Can you work these out from the model? Positions are in its coordinate system, mm. Face numbers are marked on the shaded views. Give positions to 0.01 mm unless a question says otherwise; leave off trailing zeros. Write each loop counter-clockwise with the first axis right and the second up, starting at its lowest first coordinate (ties: lowest second). Pieces come first, ordered by that corner, then holes.
1. Suppose I cut it at C-C (y = 11). Please give me the cut outline in (x, z) (1 decimal).
2. I'm going to push flat-ended pins straight in: pin 1 (12 mm diameter, centred on x = -8.5, y = -8.5, fed in from +Z); pin 2 (3 mm diameter, centred on y = 8.5, z = 13.5, fed in from -X); pin 3 (1.5 mm diameter, centred on x = 19.5, y = -7, fed in from -Z) (3 decimals). Where does each tip first touch, or does it pass through?
3. Thinking about a two-plate mould opening in X: for the marked faces 1, 2 and 3, which applies, pulls with the +X half, pulls with the -X half, needs draft (parallel to the pull), parting line crosses it, or undercut?
4. If I drill on probe 1 along Z at (x, y) = (-4, 0.75); probe 2 along X at (y, z) = (4.75, 0); probe 3 along Z at (x, y) = (-7, 7), over which ranges is the centre line in solid material (lowest first)?
5. Suppose I cut it at B-B (x = 0). Please give me the cut outline in (y, z), and give its area (3 significant figures).
6. Suppose I cut it at D-D (y = 7.75). Please give me the cut outline in (x, z) (1 decimal).
7. Suppose I cut it at A-A (z = 0). Please give me the cut outline in (x, y), and give its area (3 significant figures).
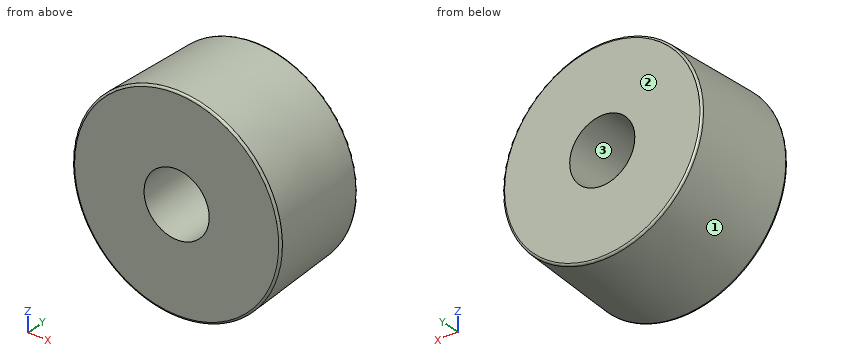
```python
from build123d import *

# Parameters (mm, degrees)
SKETCH1_R           = 25.4
SKETCH1_R_2         = 7.9375
BOSS_EXTRUDE1_DEPTH = 12.7
CHAMFER1_SIZE       = 25.4
CHAMFER1_SIZE_2     = 1.10898795
FILLET1_R           = 0.5


with BuildPart() as part:
    # Sketch1 → Boss-Extrude1 (new, symmetric)
    with BuildSketch(Plane(origin=(0, 0, 0), x_dir=(1, 0, 0), z_dir=(0, 1, 0))):
        with Locations(Location((0, 0, 0), (0, 0, 270))):
            Circle(SKETCH1_R)
        with Locations(Location((0, 0, 0), (0, 0, 270))):
            Circle(SKETCH1_R_2, mode=Mode.SUBTRACT)
    extrude(amount=BOSS_EXTRUDE1_DEPTH, both=True)

    # Chamfer1
    # the kernel refuses this chamfer: 25.4, 1.10898795 mm, written as the material it takes off along each edge
    with BuildSketch(Plane(origin=(0, 12.7, 0), x_dir=(0, 0, 1), z_dir=(-1, 0, 0))) as chamfer1_piece_1:
        Polygon((25.4, -CHAMFER1_SIZE), (25.4 - CHAMFER1_SIZE_2, 0), (25.4, 0), align=None)
    revolve(axis=Axis((0, 12.7, 0), (0, 1, 0)), mode=Mode.SUBTRACT)

    # Fillet1
    fillet1_edges = [part.edges().sort_by_distance(p)[0] for p in [
        (0, -12.7, -25.4),
        (0, 12.7, -24.29101205),
    ]]
    fillet(fillet1_edges, radius=FILLET1_R)


solid = part.part
```
Checks:
1. outline: circle Ø48.7 at (0, 0); hole circle Ø15.9 at (0, 0)
2. pin 1: stops at z = 25.14
2. pin 2: stops at x = -21.33
2. pin 3: stops at z = -16.765
3. face 1: parting line crosses it
3. face 2: needs draft
3. face 3: undercut
4. probe 1: z = -24.49 to -6.86, 6.86 to 24.49
4. probe 2: x = -24.64 to -7.94, 7.94 to 24.64
4. probe 3: z = -23.52 to -3.74, 3.74 to 23.52
5. outline: (-12.7, -24.88) arc R0.5 ccw to (-12.18, -25.38) - (12.22, -24.31) arc R0.5 ccw to (12.7, -23.81) - (12.7, -7.94) - (-12.7, -7.94) - close; (-12.7, 7.94) - (12.7, 7.94) - (12.7, 23.81) arc R0.5 ccw to (12.22, 24.31) - (-12.18, 25.38) arc R0.5 ccw to (-12.7, 24.88) - close
5. area: 859 mm2
6. outline: circle Ø49 at (0, 0); hole circle Ø15.9 at (0, 0)
7. outline: (-25.38, -12.18) arc R0.5 ccw to (-24.88, -12.7) - (-7.94, -12.7) - (-7.94, 12.7) - (-23.81, 12.7) arc R0.5 ccw to (-24.31, 12.22) - close; (7.94, -12.7) - (24.88, -12.7) arc R0.5 ccw to (25.38, -12.18) - (24.31, 12.22) arc R0.5 ccw to (23.81, 12.7) - (7.94, 12.7) - close
7. area: 859 mm2
